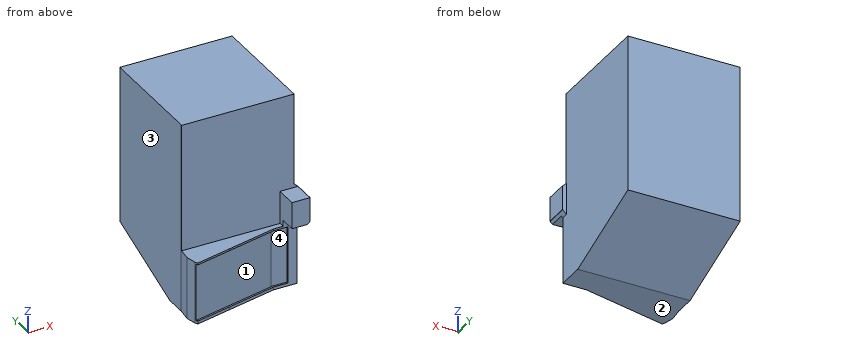
Autodesk Inventor part; units mm, degrees
ref_plane "Work Plane2" through (-266.75, -268.75, -918) normal (0, 0, -1) x (0, 1, 0)
ref_plane "YZ Plane" through (0, 0, 0) normal (1, 0, 0) x (0, 1, 0)
ref_plane "XZ Plane" through (0, 0, 0) normal (0, 1, 0) x (-1, 0, 0)
ref_plane "Work Plane1" through (0, 0, 0) normal (0, 0, 1) x (1, 0, 0)
sketch "Sketch1" plane through (0, 0, 0) normal (0, 0, 1) x (1, 0, 0)
  line L0 (271, 270) -> (271, -270)
  line L1 (-271, 270) -> (271, 270)
  line L2 (271, -273) -> (271, -270)
  line L3 (262.1457, -273) -> (289.056, -273)
  line L4 (290.5196, -278) -> (290.5196, -273)
  arc A0 (221.5544, -380.4278) -> (259.4491, -380.4278) centre (240.5018, -345.2) ccw
  line L5 (-86.5386, -360.7555) -> (157.2553, -305.3974)
  line L6 (-260.1199, -400.1704) -> (-86.5386, -360.7555)
  line L7 (-265.6803, -388.102) -> (-276.918, -338.6119)
  line L8 (-271, -270) -> (-271, 270)
  line L9 (-278.1369, -338.8887) -> (-266.8992, -388.3788)
  line L10 (-260.1199, -400.1704) -> (-266.8992, -388.3788)
  line L11 (-266.8992, -388.3788) -> (-278.1369, -338.8887)
  line L12 (-278.1369, -338.8887) -> (-271, -273)
  line L13 (-271, -273) -> (-271, 270)
  line L14 (-271, 270) -> (271, 270)
  line L15 (271, 270) -> (271, -273)
  line L16 (271, -273) -> (290.5196, -273)
  line L17 (290.5196, -273) -> (290.5196, -303.7097)
  line L18 (290.5196, -303.7097) -> (290.5196, -384.6531)
  line L19 (205.5016, -303.2) -> (205.4838, -303.7097)
  line L20 (290.5196, -384.6531) -> (202.6414, -384.6531)
  line L21 (202.6414, -305.3974) -> (202.6414, -384.6531)
  line L22 (202.6414, -305.3974) -> (157.2553, -305.3974)
  line L23 (157.2553, -305.3974) -> (-260.1199, -400.1704)
  point P0 (0, 0)
ref_plane "Work Plane2" through (-266.75, -268.75, -918) normal (0, 0, -1) x (0, 1, 0)
extrude "Extrusion1" add sketch "Sketch1" against normal up to surface (918 mm away) contours L0 L2 L3 L16 L4 L17 L18 L20 L21 L22 L5 L6 L10 L9 L12 L13 L8 L1
sketch "Sketch2" plane through (202.6414, -384.6531, 0) normal (-1, 0, 0) x (0, 0, 1)
  line L0 (0, 0) -> (0, 111.6531)
  line L1 (0, 79.2557) -> (-918, 79.2557)
  line L2 (0, 0) -> (-618, 0)
  line L3 (-618, 0) -> (-618, 79.2557)
  line L4 (-618, 79.2557) -> (0, 79.2557)
  line L5 (0, 79.2557) -> (0, 0)
  line L6 (-623, -15.5173) -> (-623, 23.8976)
  line L7 (-918, 79.2557) -> (-918, 0)
  line L8 (0, 79.2557) -> (0, 0)
  line L9 (0, 0) -> (-618, 0)
  line L10 (-618, 0) -> (-618, -151.7168)
  line L11 (-618, -151.7168) -> (0, -151.7168)
  line L12 (0, -151.7168) -> (0, 0)
  line L13 (0, 111.6531) -> (-918, 111.6531)
  line L14 (0, 79.2557) -> (-618, 79.2557)
  line L15 (-618, 79.2557) -> (-618, 106.6531)
  line L16 (-618, 106.6531) -> (0, 106.6531)
  line L17 (0, 106.6531) -> (0, 79.2557)
  point P0 (0, 384.6531)
  point P1 (-618, 0)
  point P2 (0, 106.6531)
  dimension "d2" = 300
  dimension "d5" = 300
  dimension "d18" = 5
extrude "Extrusion2" cut sketch "Sketch2" along normal through all
sketch "Sketch3" plane through (202.6414, -384.6531, 0) normal (0, -1, 0) x (1, 0, 0)
  line L0 (0, -618) -> (0, -918)
  line L1 (87.8782, 0) -> (0, 0)
  line L2 (0, 0) -> (0, -460)
  line L3 (0, -460) -> (87.8782, -460)
  line L4 (87.8782, -460) -> (87.8782, 0)
  line L5 (0, -918) -> (87.8782, -918)
  line L6 (0, 0) -> (0, -918)
  line L7 (87.8782, -918) -> (0, -918)
  line L8 (0, -918) -> (0, -588.5734)
  line L9 (0, -588.5734) -> (87.8782, -588.5734)
  line L10 (87.8782, -588.5734) -> (87.8782, -918)
  point P0 (-202.6414, 0)
  dimension "d8" = 460
extrude "Extrusion3" cut sketch "Sketch3" against normal up to surface (106.6531 mm away) contours L2 L1 L4 L3
sketch "Sketch4" plane through (271, -273, 0) normal (0, 1, 0) x (1, 0, 0)
  line L0 (19.5196, 0) -> (19.5196, 918)
  line L1 (-8.8543, 433.3976) -> (18.056, 460.3216)
  line L2 (0, 0) -> (0, 918)
  line L3 (19.5196, 0) -> (0, 0)
  line L4 (18.056, 577.2146) -> (-8.8543, 604.1385)
  line L5 (19.5196, 918) -> (0, 918)
  line L6 (19.5196, 918) -> (19.5196, 577.2146)
  line L7 (19.5196, 460) -> (19.5196, 918)
  line L8 (18.056, 577.2146) -> (19.5196, 577.2146)
  line L9 (18.056, 577.2146) -> (0, 595.2798)
  line L10 (0, 0) -> (0, 918)
  line L11 (0, 595.2798) -> (0, 918)
  line L12 (0, 918) -> (19.5196, 918)
  line L13 (18.056, 460.3216) -> (19.5196, 460.3216)
  line L14 (19.5196, 460.3216) -> (19.5196, 0)
  line L15 (19.5196, 0) -> (0, 0)
  line L16 (0, 0) -> (0, 442.2564)
  line L17 (0, 442.2564) -> (18.056, 460.3216)
  point P0 (-271, 0)
  point P1 (19.5196, 588.5734)
  point P2 (19.5196, 577.2146)
  point P3 (0, 595.2798)
extrude "Extrusion4" cut sketch "Sketch4" against normal up to surface (111.6531 mm away) contours L3 L2 L1 L13 L0 | L8 L4 L2 L5 L0
sketch "Sketch5" plane through (-260.1199, -400.1704, -918) normal (0.2214, -0.9752, 0) x (0.9752, 0.2214, 0)
  line L0 (-4, 291) -> (428, 291)
  line L1 (428, 291) -> (428, 14)
  line L2 (428, 14) -> (-4, 14)
  line L3 (-4, 14) -> (-4, 291)
  line L4 (0, 292) -> (178, 292)
  line L5 (250, 13) -> (0, 13)
  line L6 (-4, 300) -> (-4, 0)
  line L7 (428, 300) -> (428, 0)
  point P0 (342.2733, 918)
  dimension "d11" = 1
  dimension "d12" = 1
extrude "Extrusion5" cut sketch "Sketch5" against normal blind 9
sketch "Sketch6" plane through (-274.5092, -305.3974, 0) normal (0, -1, 0) x (1, 0, 0)
  line L0 (14.3893, -627) -> (431.7645, -627)
  line L1 (423.6845, -627) -> (501.5092, -627)
  line L2 (501.5092, -627) -> (501.5092, -904)
  line L3 (501.5092, -904) -> (423.6845, -904)
  line L4 (423.6845, -904) -> (423.6845, -627)
  line L5 (502.5092, -657) -> (502.5092, -620)
  line L6 (502.5092, -911) -> (502.5092, -874)
  point P0 (274.5092, 0)
  dimension "d15" = 1
extrude "Extrusion6" cut sketch "Sketch6" against normal blind 9
extrude "Extrusion7" cut sketch "Sketch3" against normal up to surface (79.2557 mm away) contours L6 L9 L10 L5 L0
sketch "Sketch7" plane through (-271, -273, 0) normal (-1, 0, 0) x (0, 0, 1)
  line L0 (-918, 543) -> (-918, 0)
  line L1 (-918, 100) -> (-758, 543)
  line L2 (0, 543) -> (-918, 543)
  line L3 (-918, 543) -> (-758, 543)
  line L4 (-918, 543) -> (-918, 100)
  point P0 (0, 273)
  dimension "d21" = 100
  dimension "d22" = 160
extrude "Extrusion8" cut sketch "Sketch7" against normal through all
equation "\"d5\" = d2"
equation "\"d12\" = d11"
properties part number "body_collisio"
Build history of the part. All positions in model axes, mm. Face numbers are marked on the shaded views. Round coordinates to 2 decimals unless told otherwise and drop trailing zeros. Write each loop counter-clockwise with the first axis right and the second up, starting at its lowest first coordinate (ties: lowest second). Pieces come first, ordered by that corner, then holes. Notation, with made-up numbers: (69.25, 2.5) -> (114.25, 2.5) arc R3 ccw to (114.25, 7.5) -> close; hole circle Ø9 at (67.5, 71). An arc over 180 degrees is marked (long way). Put each result on its own line as item: value.
Item 1: Slice it at C-C, the plane y = -224.5. Give the cut face in (x, z).
Here are the results:
outline: (-271, -918) -> (271, -918) -> (271, 0) -> (-271, 0) -> close
Item 2: Wall check: probe 1 along Y at (x, z) = (-57.5, -275); probe 2 along X at (y, z) = (220.5, -252.5); probe 3 along Y at (x, z) = (249, -524.5). Give the ranges that are in metal, low to high. Write a range as from..to.
Here are the results:
probe 1: y = -278..270
probe 2: x = -271..271
probe 3: y = -384.65..270
Item 3: Two-plate mould, pull along Z, no slides. Class the marked faces 1, 2, 3 and 4: pulls with the +Z half, pulls with the -Z half, needs draft (parallel to the pull), parting line crosses it, or undercut.
Here are the results:
face 1: undercut
face 2: pulls with the -Z half
face 3: needs draft
face 4: undercut
Item 4: Slice it at A-A, the plane z = -510.5. Give the cut face in (x, y), plus the area to 3 significant figures.
Here are the results:
outline: (-271.54, -278) -> (202.64, -278) -> (202.64, -384.65) -> (290.52, -384.65) -> (290.52, -273) -> (271, -273) -> (271, 270) -> (-271, 270) -> (-271, -273) -> close
area: 306,000 mm^2
Item 5: Slice it at D-D, the plane z = -653. Give the cut face in (x, y), plus the area to 3 significant figures.
Here are the results:
outline: (-278.14, -338.89) -> (-266.9, -388.38) -> (-264.81, -392.01) -> (149.18, -298.02) -> (149.18, -296.4) -> (227, -296.4) -> (227, -305.4) -> (271, -305.4) -> (271, 270) -> (-271, 270) -> (-271, -273) -> close
area: 328,000 mm^2
Item 6: Flat gauge pins, fed straight in: P1, Ø10, axis at y = -302.5, z = -738.5, coming from the -X side; P2, Ø1.6, axis at x = 290, y = -355, coming from the -Z side; P3, Ø1.3, axis at y = -297.5, z = -777.5, coming from the +X side. Where does each tip first touch, or does it go through?
Here are the results:
P1: stops at x = -274.74
P2: stops at z = -577.21
P3: stops at x = 271
Item 7: Slice it at B-B, the plane x = -109. Give the cut face in (y, z), plus the area to 3 significant figures.
Here are the results:
outline: (-365.86, -918) -> (-173, -918) -> (270, -758) -> (270, 0) -> (-278, 0) -> (-278, -618) -> (-365.86, -618) -> (-365.86, -627) -> (-356.63, -627) -> (-356.63, -904) -> (-365.86, -904) -> close
area: 491,000 mm^2
